Check sheet for the modelled part. Datum: model origin and axes. Units: mm. A direction names the side the tool comes from. Round coordinates to 2 decimals unless told otherwise and drop trailing zeros. Order: outer loops, then holes, each group sorted by start corner. A loop starts at its lowest first (then second) coordinate and runs counter-clockwise, first axis right, second up.
```python
from build123d import *

# Parameters (mm, degrees)
SKETCH1_R           = 40
BOSS_EXTRUDE1_DEPTH = 10
SKETCH2_R           = 10
BOSS_EXTRUDE2_DEPTH = 550
SKETCH3_R           = 10
BOSS_EXTRUDE3_DEPTH = 30


with BuildPart() as part:
    # Sketch1 → Boss-Extrude1 (new body)
    with BuildSketch(Plane.XY):
        Circle(SKETCH1_R)
    extrude(amount=BOSS_EXTRUDE1_DEPTH)

    # Sketch2 → Boss-Extrude2 (add)
    with BuildSketch(Plane.XY.offset(10)):
        Circle(SKETCH2_R)
    extrude(amount=BOSS_EXTRUDE2_DEPTH)

    # Sketch3 → Boss-Extrude3 (add)
    with BuildSketch(Plane(origin=(0, 0, 0), x_dir=(-1, 0, 0), z_dir=(0, 0, -1))):
        with Locations((26.998561916, 0)):
            Circle(SKETCH3_R)
    extrude(amount=BOSS_EXTRUDE3_DEPTH)


solid = part.part
```
Item 1: Sectioned sample at B-B (x = 0). Record the cut outline in (y, z), and give its area (3 significant figures).
Answer:
outline: (-40, 0) - (40, 0) - (40, 10) - (10, 10) - (10, 560) - (-10, 560) - (-10, 10) - (-40, 10) - close
area: 11,800 mm2
Item 2: Sectioned sample at D-D (y = -26). Record the cut outline in (x, z), and give its area (3 significant figures).
Answer:
outline: (-30.4, 0) - (30.4, 0) - (30.4, 10) - (-30.4, 10) - close
area: 608 mm2
Item 3: Go/stop test with flat-tipped pins: P1, Ø4, axis at x = -23.5, y = 26, coming from the +Z side; P2, Ø1, axis at y = -7, z = 88, coming from the -X side; P3, Ø3, axis at x = 2, z = 263.5, coming from the +Y side. Record where each tip stops, or that it passes through.
Answer:
P1: stops at z = 10
P2: stops at x = -7.6
P3: stops at y = 9.99
Item 4: Sectioned sample at C-C (z = 147.5). Record the cut outline in (x, y).
Answer:
outline: circle Ø20 at (0, 0)
Item 5: Sectioned sample at A-A (y = 0). Record the cut outline in (x, z), and give its area (3 significant figures).
Answer:
outline: (-40, 0) - (-37, 0) - (-37, -30) - (-17, -30) - (-17, 0) - (40, 0) - (40, 10) - (10, 10) - (10, 560) - (-10, 560) - (-10, 10) - (-40, 10) - close
area: 12,400 mm2
Item 6: Access from +Z, -Z, +X, -X, +Y, -Y to the whole of each face (thin tool, end or side, straight path). Record for faces 1 (the flat face through (0, 0, 560)), 2 (the cylindrical face through (-2.17, -9.76, 281.15)), 3 (the cylindrical face through (-36.54, 3, -14.79)).
Answer:
face 1: +Z, +X, -X, +Y, -Y
face 2: +Z
face 3: -Z
Item 7: Scan lines: line 1 along Z through (x, y) = (14, -14.5); line 2 along X through (y, z) = (-0.5, 428.5); line 3 along Z through (x, y) = (-6, -4.5). Record each from-to range of solid material in increasing order.
Answer:
line 1: z = 0 to 10
line 2: x = -9.99 to 9.99
line 3: z = 0 to 560
